For this review, take the finished solid that the model builds, in its own axes (mm). Give positions to 0.01 mm unless a question says otherwise; leave off trailing zeros. Loops run counter-clockwise (first coordinate to the right, second up) from the corner with the lowest first, then second, coordinate; pieces in that order, holes last. Notation, with made-up numbers: (7, 89) - (30, 89) arc R12 cw to (30, 95) - close; hole circle Ø2 at (-17.5, 61). An arc over 180 degrees is marked (long way). Use CSV: the item, a comma, the result in double quotes. Start each with the question number.
1. Take a section at C-C on x = 326.5. Give the boundary of the cut face in (y, z), plus the area to 4 significant figures.
2. Wall thickness on line 1 (X direction, y = 190, z = 4.1); line 2 (X direction, y = 287, z = 1.35); line 3 (Y direction, x = 272, z = 4.3): over which ranges is each line inside the solid? List them lowest first.
3. Take a section at B-B on y = 312.5. Give the boundary of the cut face in (x, z), plus the area to 4 significant figures.
4. Take a section at A-A on z = 2.55. Give the boundary of the cut face in (x, y) (3 decimals), plus the area to 3 significant figures.
5. For pin 1 (1.5 mm diameter, centred on x = 299.5, z = 3.5, fed in from +Y), flat-tipped, find the tip position at first contact; note if it passes through.
```python
from build123d import *

# Parameters (mm, degrees)
SKETCH1_W           = 540
SKETCH1_H           = 540
BOSS_EXTRUDE1_DEPTH = 5
CHAMFER2_SIZE       = 0.5
CHAMFER3_SIZE       = 2
SKETCH3_W           = 150
SKETCH3_H           = 20
CUT_EXTRUDE2_DEPTH  = 10
CIRPATTERN1_COUNT   = 4
CUT_EXTRUDE3_DEPTH  = 10
LPATTERN1_COUNT     = 2
LPATTERN1_PITCH     = 32.5
LPATTERN2_COUNT     = 2
LPATTERN2_PITCH     = 32.5
SKETCH7_W           = 697.267045649
SKETCH7_H           = 709.774077858
SKETCH7_W_2         = 250
SKETCH7_H_2         = 539
CUT_EXTRUDE4_DEPTH  = 764.691691719


with BuildPart() as part:
    # Sketch1 → Boss-Extrude1 (new body)
    with BuildSketch(Plane.XY):
        with Locations((270, 270)):
            Rectangle(SKETCH1_W, SKETCH1_H)
    extrude(amount=BOSS_EXTRUDE1_DEPTH)

    # Chamfer2
    chamfer2_edges = [part.edges().sort_by_distance(p)[0] for p in [
        (540, 270, 5),
        (270, 540, 5),
        (0, 270, 5),
        (270, 540, 0),
        (540, 270, 0),
        (270, 0, 0),
        (0, 270, 0),
        (270, 0, 5),
    ]]
    chamfer(chamfer2_edges, length=CHAMFER2_SIZE)

    # Chamfer3
    # the kernel refuses this chamfer: 2 mm, written as the material it takes off along each edge
    with BuildSketch(Plane(origin=(0, 540, -4.643365976), x_dir=(-0.027495876610586483, -0.9996219169112968, 0), z_dir=(0, 0, 1)), Plane(origin=(0, 0, -4.643365976), x_dir=(0.9996219169112968, -0.027495876610586372, 0), z_dir=(0, 0, 1))) as chamfer3_piece_1:
        Polygon((CHAMFER3_SIZE * 0.999621916911, CHAMFER3_SIZE * 0.0274958766106), (-CHAMFER3_SIZE * 0.0274958766106, CHAMFER3_SIZE * 0.999621916911), (0, 0), align=None)
    extrude(amount=14.286731952, mode=Mode.SUBTRACT)
    with BuildSketch(Plane(origin=(540, 540, -4.643365976), x_dir=(0.02749587661058229, -0.9996219169112968, 0), z_dir=(0, 0, 1)), Plane(origin=(540, 0, -4.643365976), x_dir=(-0.9996219169112968, -0.027495876610586483, 0), z_dir=(0, 0, 1))) as chamfer3_piece_2:
        Polygon((CHAMFER3_SIZE * 0.999621916911, -CHAMFER3_SIZE * 0.0274958766106), (-CHAMFER3_SIZE * 0.0274958766106, -CHAMFER3_SIZE * 0.999621916911), (0, 0), align=None)
    extrude(amount=14.286731952, mode=Mode.SUBTRACT)

    # Sketch3 → Cut-Extrude2 (cut)
    with BuildSketch(Plane.XY.offset(5)):
        with Locations((270, 530)):
            Rectangle(SKETCH3_W, SKETCH3_H)
    cut_extrude2 = extrude(amount=-CUT_EXTRUDE2_DEPTH, mode=Mode.SUBTRACT)

    # CirPattern1: Cut-Extrude2 ×4 about axis
    cirpattern1_axis = Axis((270.5, 269.5, 0), (0, 0, 1))
    for i in range(1, CIRPATTERN1_COUNT):
        add(cut_extrude2.rotate(cirpattern1_axis, i * 360 / CIRPATTERN1_COUNT), mode=Mode.SUBTRACT)

    # Sketch6 → Cut-Extrude3 (cut)
    with BuildSketch(Plane.XY.offset(5)):
        with BuildLine():
            Line((272.800394222, 369.50499001), (273.199595818, 169.50499001))
            ThreePointArc((273.199595818, 169.50499001), (270.704590808, 167.00000498), (268.199605778, 169.49500999))
            Line((268.199605778, 169.49500999), (267.800404182, 369.49500999))
            ThreePointArc((267.800404182, 369.49500999), (270.295409192, 371.99999502), (272.800394222, 369.50499001))
        make_face()
    cut_extrude3 = extrude(amount=-CUT_EXTRUDE3_DEPTH, mode=Mode.SUBTRACT)

    # LPattern1: Cut-Extrude3 ×2
    with Locations(*[(i * LPATTERN1_PITCH, 0, 0) for i in range(1, LPATTERN1_COUNT)]):
        add(cut_extrude3, mode=Mode.SUBTRACT)

    # LPattern2: Cut-Extrude3 ×2
    with Locations(*[(-i * LPATTERN2_PITCH, 0, 0) for i in range(1, LPATTERN2_COUNT)]):
        add(cut_extrude3, mode=Mode.SUBTRACT)

    # Sketch7 → Cut-Extrude4 (cut, through all)
    with BuildSketch(Plane.XY.offset(5)):
        with Locations((264.820460551, 266.911861518)):
            Rectangle(SKETCH7_W, SKETCH7_H)
        with Locations((270.5, 270)):
            Rectangle(SKETCH7_W_2, SKETCH7_H_2, mode=Mode.SUBTRACT)
    extrude(amount=-CUT_EXTRUDE4_DEPTH, mode=Mode.SUBTRACT)


solid = part.part
```
Check result:
1,outline,"(19, 0) - (520, 0) - (520, 5) - (19, 5) - close"
1,area,"2,505 mm²"
2,line 1,"x = 145.5 to 235.66, 240.66 to 268.16, 273.16 to 300.66, 305.66 to 395.5"
2,line 2,"x = 145.5 to 235.47, 240.47 to 267.97, 272.97 to 300.47, 305.47 to 395.5"
2,line 3,"y = 19 to 167.36, 371.33 to 520"
3,outline,"(145.5, 0) - (235.41, 0) - (235.41, 5) - (145.5, 5) - close; (240.41, 0) - (267.91, 0) - (267.91, 5) - (240.41, 5) - close; (272.91, 0) - (300.41, 0) - (300.41, 5) - (272.91, 5) - close; (305.41, 0) - (395.5, 0) - (395.5, 5) - (305.41, 5) - close"
3,area,"1,175 mm²"
4,outline,"(145.5, 0.5) - (196, 0.5) - (196, 19) - (346, 19) - (346, 0.5) - (395.5, 0.5) - (395.5, 539.5) - (345, 539.5) - (345, 520) - (195, 520) - (195, 539.5) - (145.5, 539.5) - close; hole (235.3, 369.495) - (235.7, 169.495) arc R2.5 ccw to (240.7, 169.505) - (240.3, 369.505) arc R2.5 ccw to start; hole (267.8, 369.495) - (268.2, 169.495) arc R2.5 ccw to (273.2, 169.505) - (272.8, 369.505) arc R2.5 ccw to start; hole (300.3, 369.495) - (300.7, 169.495) arc R2.5 ccw to (305.7, 169.505) - (305.3, 369.505) arc R2.5 ccw to start"
4,area,"126,000 mm²"
5,pin 1,"stops at y = 520"
